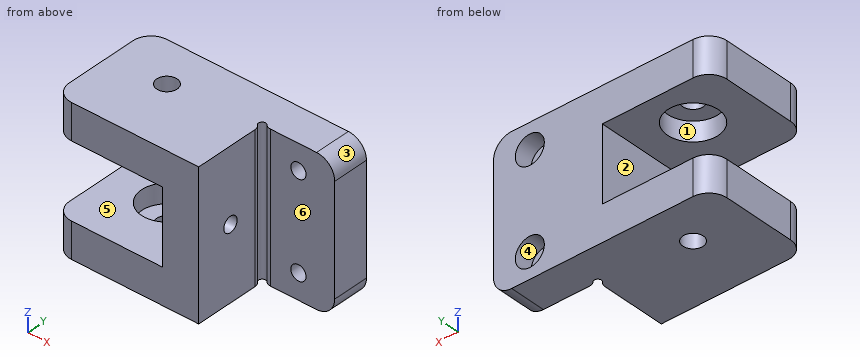
from build123d import *

# Parameters (mm, degrees)
DODANIE_WYCI_GNI_CIE1_DEPTH = 40
SZKIC4_W                    = 9.8
SZKIC4_H                    = 30
DODANIE_WYCI_GNI_CIE3_DEPTH = 30
SZKIC6_R                    = 7
WYTNIJ_WYCI_GNI_CIE1_DEPTH  = 65.031242374
SZKIC7_R                    = 4
WYTNIJ_WYCI_GNI_CIE2_DEPTH  = 5
SZKIC8_R                    = 2.1
WYTNIJ_WYCI_GNI_CIE3_DEPTH  = 5
SZKIC9_R                    = 4
WYTNIJ_WYCI_GNI_CIE4_DEPTH  = 5
SZKIC10_R                   = 2.1
WYTNIJ_WYCI_GNI_CIE5_DEPTH  = 5
ZAOKR_GLENIE1_R             = 5
ZAOKR_GLENIE2_R             = 5
SZKIC11_R                   = 7
DODANIE_WYCI_GNI_CIE5_DEPTH = 4.5
SZKIC12_R                   = 2.8
WYTNIJ_WYCI_GNI_CIE6_DEPTH  = 65.031242374


with BuildPart() as part:
    # Szkic1 → Dodanie-wyciągnięcie1 (new body)
    with BuildSketch(Plane.XY):
        with BuildLine():
            Line((0, 0), (0, 17.763932023))
            ThreePointArc((0, 17.763932023), (-0.174258142, 18.580428603), (-0.666666667, 19.254644008))
            ThreePointArc((-0.666666667, 19.254644008), (-0.707106781, 20.707106781), (0.745355992, 20.666666667))
            ThreePointArc((0.745355992, 20.666666667), (1.419571397, 20.174258142), (2.236067977, 20))
            Line((2.236067977, 20), (20, 20))
            Line((20, 20), (20, 30))
            Line((20, 30), (-10, 30))
            Line((-10, 30), (-10, 0))
            Line((-10, 0), (0, 0))
        make_face()
    extrude(amount=DODANIE_WYCI_GNI_CIE1_DEPTH)

    # Szkic4 → Dodanie-wyciągnięcie3 (add)
    with BuildSketch(Plane.ZY.offset(10)):
        with Locations((35.1, 15)):
            Rectangle(SZKIC4_W, SZKIC4_H)
        with Locations((4.9, 15)):
            Rectangle(SZKIC4_W, SZKIC4_H)
    extrude(amount=DODANIE_WYCI_GNI_CIE3_DEPTH)

    # Szkic6 → Wytnij-wyciągnięcie1 (cut, through all)
    with BuildSketch(Plane.XY.offset(40)):
        with Locations((-24.5, 18)):
            Circle(SZKIC6_R)
    extrude(amount=-WYTNIJ_WYCI_GNI_CIE1_DEPTH, mode=Mode.SUBTRACT)

    # Szkic7 → Wytnij-wyciągnięcie2 (cut)
    with BuildSketch(Plane.ZY.offset(10)):
        with Locations(Location((20, 10, 0), (0, 0, 270))):
            Circle(SZKIC7_R)
    extrude(amount=-WYTNIJ_WYCI_GNI_CIE2_DEPTH, mode=Mode.SUBTRACT)

    # Szkic8 → Wytnij-wyciągnięcie3 (cut)
    with BuildSketch(Plane.ZY.offset(5)):
        with Locations(Location((20, 10, 0), (0, 0, 270))):
            Circle(SZKIC8_R)
    extrude(amount=-WYTNIJ_WYCI_GNI_CIE3_DEPTH, mode=Mode.SUBTRACT)

    # Szkic9 → Wytnij-wyciągnięcie4 (cut)
    with BuildSketch(Plane(origin=(0, 30, 0), x_dir=(1, 0, 0), z_dir=(0, 1, 0))):
        with Locations(Location((10, -33, 0), (0, 0, 180))):
            Circle(SZKIC9_R)
        with Locations(Location((10, -7, 0), (0, 0, 180))):
            Circle(SZKIC9_R)
    extrude(amount=-WYTNIJ_WYCI_GNI_CIE4_DEPTH, mode=Mode.SUBTRACT)

    # Szkic10 → Wytnij-wyciągnięcie5 (cut)
    with BuildSketch(Plane(origin=(0, 25, 0), x_dir=(1, 0, 0), z_dir=(0, 1, 0))):
        with Locations(Location((10, -33, 0), (0, 0, 180))):
            Circle(SZKIC10_R)
        with Locations(Location((10, -7, 0), (0, 0, 180))):
            Circle(SZKIC10_R)
    extrude(amount=-WYTNIJ_WYCI_GNI_CIE5_DEPTH, mode=Mode.SUBTRACT)

    # Zaokrąglenie1
    zaokr_glenie1_edges = [part.edges().sort_by_distance(p)[0] for p in [
        (20, 25, 0),
        (20, 25, 40),
    ]]
    fillet(zaokr_glenie1_edges, radius=ZAOKR_GLENIE1_R)

    # Zaokrąglenie2
    zaokr_glenie2_edges = [part.edges().sort_by_distance(p)[0] for p in [
        (-40, 30, 35.1),
        (-40, 0, 35.1),
        (-40, 0, 4.9),
        (-40, 30, 4.9),
    ]]
    fillet(zaokr_glenie2_edges, radius=ZAOKR_GLENIE2_R)

    # Szkic11 → Dodanie-wyciągnięcie5 (add)
    with BuildSketch(Plane.XY.offset(40)):
        with Locations((-24.5, 18)):
            Circle(SZKIC11_R)
    dodanie_wyci_gni_cie5 = extrude(amount=-DODANIE_WYCI_GNI_CIE5_DEPTH)

    # Lustro1: Dodanie-wyciągnięcie5 across plane
    add(dodanie_wyci_gni_cie5.mirror(Plane.XY.offset(20)))

    # Szkic12 → Wytnij-wyciągnięcie6 (cut, through all)
    with BuildSketch(Plane.XY.offset(40)):
        with Locations((-24.5, 18)):
            Circle(SZKIC12_R)
    extrude(amount=-WYTNIJ_WYCI_GNI_CIE6_DEPTH, mode=Mode.SUBTRACT)


solid = part.part
Build history of the part. All positions in model axes, mm. Face numbers are marked on the shaded views. A direction names the side the tool comes from. Coordinates: 2 decimals unless noted, no trailing zeros. Order: outer loops, then holes, each group sorted by start corner. A loop starts at its lowest first (then second) coordinate and runs counter-clockwise, first axis right, second up. Notation, with made-up numbers: (58, -35.5) - (111, -35.5) arc R7 cw to (111, -26.5) - close; hole circle Ø11 at (9, 77.25). An arc over 180 degrees is marked (long way). Write each question's results on one line, items separated by ' | '. Start each with the question number.
Item 1: Band-saw the part on D-D on x = -8. Write the cut outline in (y, z), and give its area (3 significant figures).
Item 2: Wall check: probe 1 along Z at (x, y) = (10, 27.8); probe 2 along Z at (x, y) = (-16.5, 21.25); probe 3 along Y at (x, z) = (-24.5, 2.6). Give the ranges that are in metal, low to high. Write a range as [from, to].
Item 3: Tool access for the marked faces 4, 5 and 6: list every direction of +Z, -Z, +X, -X, +Y, -Y with a clear straight run to the whole face (end or side of a thin tool).
Item 4: Band-saw the part on C-C on z = 33. Write the cut outline in (x, y), and give its area (3 significant figures).
Item 5: Flat gauge pins, fed straight in: pin 1 (12 mm diameter, centred on y = 12, z = 23, fed in from +X); pin 2 (6.5 mm diameter, centred on x = 10, z = 33, fed in from -Y); pin 3 (9 mm diameter, centred on y = 9.5, z = 20.5, fed in from -X). Where does each tip first touch, or does it go through?
Item 6: Band-saw the part on B-B on x = -24.5. Write the cut outline in (y, z).
Item 7: Mould opens along X. For the marked faces 1, 2 and 3 say: released by +X, released by -X, zero draft, split by the parting line, or undercut.
Item 8: Band-saw the part on A-A on z = 20. Write the cut outline in (x, y).
Numbers:
1) outline: (0, 0) - (30, 0) - (30, 40) - (0, 40) - close; hole circle Ø8 at (10, 20) | area: 1,150 mm^2
2) probe 1: [0, 3], [11, 29], [37, 40] | probe 2: [0, 9.8], [30.2, 40] | probe 3: [0, 15.2], [20.8, 30]
3) face 4: +Y | face 5: -X, +Y, -Y | face 6: +Z, -Z, +X, -Y
4) outline: (-40, 5) arc R5 ccw to (-35, 0) - (0, 0) - (0, 17.76) arc R2 ccw to (-0.67, 19.25) arc R1 cw (long way) to (0.75, 20.67) arc R2 ccw to (2.24, 20) - (7.9, 20) - (7.9, 25) - (6, 25) - (6, 30) - (-35, 30) arc R5 ccw to (-40, 25) - close; (12.1, 20) - (20, 20) - (20, 30) - (14, 30) - (14, 25) - (12.1, 25) - close; hole circle Ø14 at (-24.5, 18) | area: 1,170 mm^2
5) pin 1: x = 0 | pin 2: y = 20 | pin 3: x = -10
6) outline: (0, 0) - (15.2, 0) - (15.2, 4.5) - (11, 4.5) - (11, 9.8) - (0, 9.8) - close; (0, 30.2) - (11, 30.2) - (11, 35.5) - (15.2, 35.5) - (15.2, 40) - (0, 40) - close; (20.8, 0) - (30, 0) - (30, 9.8) - (25, 9.8) - (25, 4.5) - (20.8, 4.5) - close; (20.8, 35.5) - (25, 35.5) - (25, 30.2) - (30, 30.2) - (30, 40) - (20.8, 40) - close
7) face 1: undercut | face 2: released by -X | face 3: released by +X
8) outline: (-10, 0) - (0, 0) - (0, 7.9) - (-5, 7.9) - (-5, 6) - (-10, 6) - close; (-10, 14) - (-5, 14) - (-5, 12.1) - (0, 12.1) - (0, 17.76) arc R2 ccw to (-0.67, 19.25) arc R1 cw (long way) to (0.75, 20.67) arc R2 ccw to (2.24, 20) - (20, 20) - (20, 30) - (-10, 30) - close
